Here's how the part is built. I have some questions about the finished solid (model axes, mm). A direction names the side the tool comes from. Round coordinates to 2 decimals unless told otherwise and drop trailing zeros. Put each result on its own line as item: value. Start each with the question number.
1) Will this pin go through, and if not, where does the flat tip stop? P1, Ø1, axis at y = 21.5, z = 2, coming from the +X side.
2) I want a section at A-A, the plane x = -11. Give the number of separate pieces and of enclosed holes in the cut face, then the cut area to 3 significant figures.
3) Which directions (+Z, -Z, +X, -X, +Y, -Y) give clear straight access to the entire face, cutting with the end or side of a thin tool? Please do faces 1 (the flat face through (7.32, -15.95, 1.61)), 2 (the flat face through (19.05, 0, 2)), 3 (the flat face through (-15.83, 7.2, 1.61)).
4) We'd pull the mould along X, two halves only. Please class faces 4 (the flat face through (-6.5, 0.2, 3.175)), 5 (the flat face through (1.61, -25.31, 1.57)), 6 (the flat face through (-31.02, -6.18, 1.61)): released by +X, released by -X, zero draft, split by the parting line, or undercut.
5) If I drill on line 1 along X through (y, z) = (27, 2.3); line 2 along Y through (x, z) = (-27.5, 2.2); line 3 along X through (y, z) = (-24, 1.95), over which ranges is the centre line in solid material (lowest first)? Write a range as [from, to].
from build123d import *

# Parameters (mm, degrees)
F0_R     = 6.35
F1_DEPTH = 3.175
F2_SIZE  = 3.17499


# Not quite as in the source:
# - a fillet or chamfer is up to 0.001 mm smaller than in the source, because OpenCascade refuses the exact size


with BuildPart() as f1:
    # F0 (on Top) → F1 (new body)
    with BuildSketch(Plane.XY):
        Polygon((6.35, -12.6999929847), (-6.35, -12.6999929847), (-12.6999929847, -19.0499859695), (0, -50.7999929847), (12.6999929847, -19.0499859695), align=None)
        Polygon((-3.175, -19.0499929847), (3.175, -19.0499929847), (0, -31.7499929847), align=None, mode=Mode.SUBTRACT)
        Polygon((19.0499859695, 12.6999929847), (12.6999929847, 6.35), (12.6999929847, -6.35), (19.0499859695, -12.6999929847), (50.7999929847, 0), align=None)
        Polygon((19.0499929847, -3.175), (19.0499929847, 3.175), (31.7499929847, 0), align=None, mode=Mode.SUBTRACT)
        Polygon((-6.35, 12.6999929847), (-12.6999929847, 6.35), (-12.6999929847, -6.35), (-6.35, -12.6999929847), (6.35, -12.6999929847), (12.6999929847, -6.35), (12.6999929847, 6.35), (6.35, 12.6999929847), align=None)
        Circle(F0_R, mode=Mode.SUBTRACT)
        Polygon((-12.6999929847, -6.35), (-12.6999929847, 6.35), (-19.0499859695, 12.6999929847), (-50.7999929847, 0), (-19.0499859695, -12.6999929847), align=None)
        Polygon((-19.0499929847, 3.175), (-19.0499929847, -3.175), (-31.7499929847, 0), align=None, mode=Mode.SUBTRACT)
        Polygon((-12.6999929847, 19.0499859695), (-6.35, 12.6999929847), (6.35, 12.6999929847), (12.6999929847, 19.0499859695), (0, 50.7999929847), align=None)
        Polygon((3.175, 19.0499929847), (-3.175, 19.0499929847), (0, 31.7499929847), align=None, mode=Mode.SUBTRACT)
    extrude(amount=F1_DEPTH)

    # F2 (size 3.175 in the source; OpenCascade refuses exactly that, so slightly less here)
    f2_edges = [f1.edges().sort_by_distance(p)[0] for p in [
        (6.349996, -34.924989, 3.175),
        (-6.349996, -34.924989, 3.175),
        (-9.524996, -15.874989, 3.175),
        (9.524996, -15.874989, 3.175),
        (34.924989, -6.349996, 3.175),
        (15.874989, -9.524996, 3.175),
        (34.924989, 6.349996, 3.175),
        (15.874989, 9.524996, 3.175),
        (9.524996, -9.524996, 3.175),
        (-9.524996, -9.524996, 3.175),
        (-15.874989, -9.524996, 3.175),
        (-34.924989, -6.349996, 3.175),
        (-34.924989, 6.349996, 3.175),
        (-15.874989, 9.524996, 3.175),
        (-9.524996, 9.524996, 3.175),
        (9.524996, 9.524996, 3.175),
        (-9.524996, 15.874989, 3.175),
        (-6.349996, 34.924989, 3.175),
        (6.349996, 34.924989, 3.175),
        (9.524996, 15.874989, 3.175),
    ]]
    chamfer(f2_edges, length=F2_SIZE)


solid = f1.part
Findings:
1. P1: stops at x = 10.14
2. separate pieces: 3
2. enclosed holes: 0
2. area: 45.5 mm2
3. face 1: +Z, +X
3. face 2: +Z, -Z
3. face 3: +Z, +Y
4. face 4: zero draft
4. face 5: undercut
4. face 6: released by -X
5. line 1: x = [-7.04, -1.19], [1.19, 7.04]
5. line 2: y = [-6.95, -1.06], [1.06, 6.95]
5. line 3: x = [-8.62, -1.94], [1.94, 8.62]
